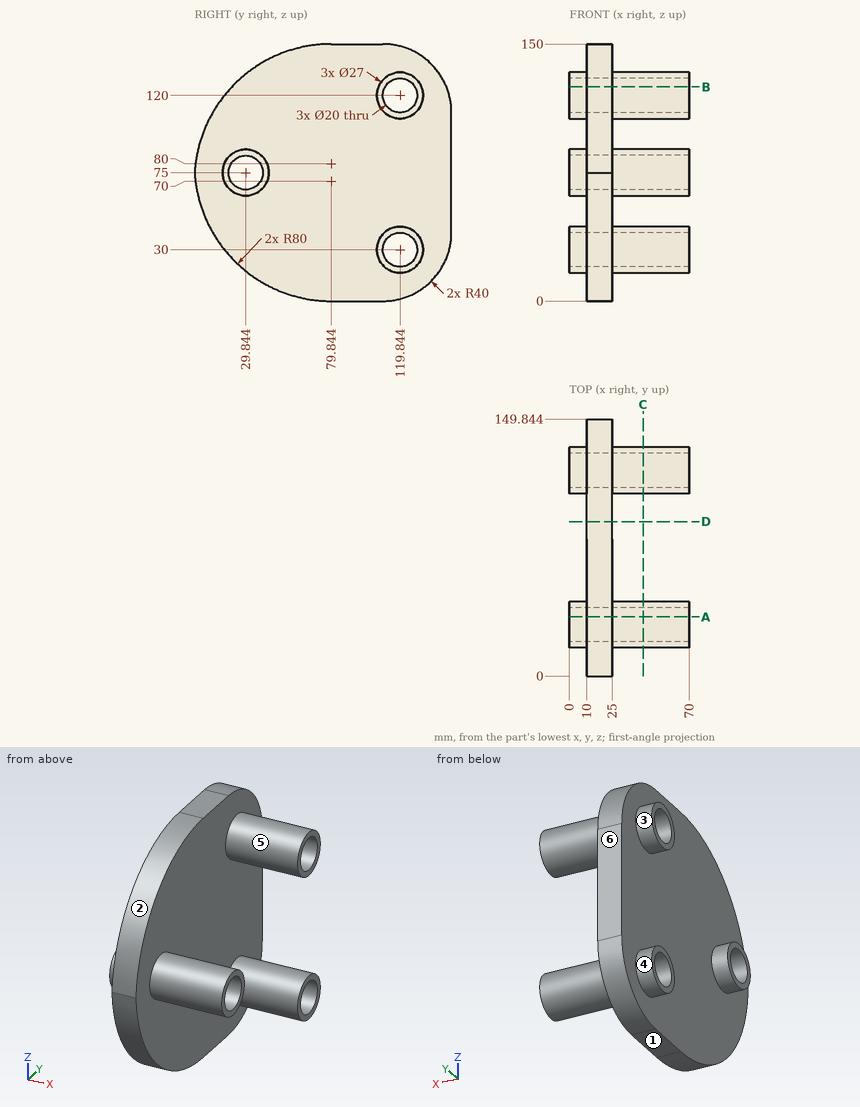
Here's the drawing with two shaded views (mm, measured from the low corner). I have some questions. A direction names the side the tool comes from. Coordinates: 2 decimals unless noted, no trailing zeros. Loops run counter-clockwise (first coordinate to the right, second up) from the corner with the lowest first, then second, coordinate; pieces in that order, holes last. Notation, with made-up numbers: M 44,-9.75 L 100,-9.75 A36 ccw 100,27.25 Z; hole C 27,42.5 d7. An arc over 180 degrees is marked long. Return JSON: item names as keys, results as strings. Group by question number.
Item 1: If I drill on L1, parallel to Y at x = 33, z = 30; L2, parallel to Z at x = 15.5, y = 124.5; L3, parallel to Z at x = 55, y = 122.5 (1 decimal), over which ranges is the centre line in solid material (lowest first)? Write a range as from..to.
Item 2: Imagine slicing it at C-C (x = 43). Please give me the cut outline in (y, z).
Item 3: Thinking about a two-plate mould opening in Z: for the marked faces 1, 2 and 3, which applies, released by +Z, released by -Z, zero draft, split by the parting line, or undercut?
Item 4: Imagine slicing it at A-A (y = 34.5). Please give me the cut outline in (x, z), and give its area (3 significant figures).
Item 5: I'm going to push flat-ended pins straight in: pin 1 Ø10 at (y, z) = (17.5, 23) entering from +X; pin 2 Ø5 at (y, z) = (54, 108.5) entering from -X; pin 3 Ø12 at (x, z) = (57.5, 64.5) entering from +Y; pin 4 Ø16 at (y, z) = (119.84, 30) entering from +X. Where does each tip first touch, or does it pass through?
Item 6: On a 3-axis mill with a long thin cutter (end or side, diameter ignored), from which of +Z, -Z, +X, -X, +Y, -Y can I reach the whole of each face in a straight line? I mean the marked faces 4, 5 and 6. Say none if no direction works.
Item 7: Imagine slicing it at D-D (y = 90). Please give me the cut outline in (x, z), and give its area (3 significant figures).
Item 8: Imagine slicing it at B-B (z = 125). Please give me the cut outline in (x, y) (1 decimal).
Verdict:
{
 "1": {"L1": "y = 106.34..109.84, 129.84..133.34", "L2": "z = 2.78..21.15, 38.85..111.15, 128.85..147.22", "L3": "z = 16.8..20.4, 39.6..43.2, 106.8..110.4, 129.6..133.2"},
 "2": {"outline": "C 29.84,75 d27; C 119.84,30 d27; C 119.84,120 d27; hole C 29.84,75 d20; hole C 119.84,30 d20; hole C 119.84,120 d20"},
 "3": {"face 1": "released by -Z", "face 2": "released by +Z", "face 3": "undercut"},
 "4": {"outline": "M 0,62.33 L 10,62.33 L 10,14.09 L 25,14.09 L 25,62.33 L 70,62.33 L 70,66.15 L 0,66.15 Z; M 0,83.85 L 70,83.85 L 70,87.67 L 25,87.67 L 25,135.91 L 10,135.91 L 10,87.67 L 0,87.67 Z", "area": "1,980 mm^2"},
 "5": {"pin 1": "stops at x = 25", "pin 2": "stops at x = 10", "pin 3": "stops at y = 42.57", "pin 4": "passes through"},
 "6": {"face 4": "-X", "face 5": "+X", "face 6": "+Z, -Z, +X, -X, +Y"},
 "7": {"outline": "M 10,0 L 25,0 L 25,150 L 10,150 Z", "area": "2,250 mm^2"},
 "8": {"outline": "M 0,107.3 L 10,107.3 L 10,21.7 L 25,21.7 L 25,107.3 L 70,107.3 L 70,111.2 L 0,111.2 Z; M 0,128.5 L 70,128.5 L 70,132.4 L 25,132.4 L 25,146.9 L 10,146.9 L 10,132.4 L 0,132.4 Z"}
}
